Read the model definition and answer for the solid it produces. Units are mm, in the model's axes. A direction names the side the tool comes from. Coordinates: 2 decimals unless noted, no trailing zeros. Order: outer loops, then holes, each group sorted by start corner. A loop starts at its lowest first (then second) coordinate and runs counter-clockwise, first axis right, second up. Notation, with made-up numbers: (49, 27.5) -> (94, 27.5) arc R29 ccw to (94, 53.5) -> close; hole circle Ø10 at (1, 26). An arc over 180 degrees is marked (long way). Use CSV: the item, a comma, the result in double quotes.
```python
from build123d import *

# Parameters (mm, degrees)
SKETCH2_W                   = 38.65
SKETCH2_H                   = 38.65
BOSS_EXTRUDE1_DEPTH         = 1.5875
SKETCH8_W                   = 7.040833333
SKETCH8_H                   = 3.175
BOSS_EXTRUDE3_DEPTH         = 3.175
LPATTERN3_COUNT             = 3
LPATTERN3_PITCH             = 13.941666667
CIRPATTERN1_COUNT           = 4
CIRPATTERN1_COPY_1_SKETCH_W = 7.040833333
CIRPATTERN1_COPY_1_SKETCH_H = 3.175
CIRPATTERN1_COPY_1_DEPTH    = 3.175
CIRPATTERN1_COPY_2_SKETCH_W = 7.040833333
CIRPATTERN1_COPY_2_SKETCH_H = 3.175
CIRPATTERN1_COPY_2_DEPTH    = 3.175
CIRPATTERN1_COPY_3_SKETCH_W = 7.040833333
CIRPATTERN1_COPY_3_SKETCH_H = 3.175
CIRPATTERN1_COPY_3_DEPTH    = 3.175
CIRPATTERN1_COPY_4_SKETCH_W = 7.040833333
CIRPATTERN1_COPY_4_SKETCH_H = 3.175
CIRPATTERN1_COPY_4_DEPTH    = 3.175
CIRPATTERN1_COPY_5_SKETCH_W = 7.040833333
CIRPATTERN1_COPY_5_SKETCH_H = 3.175
CIRPATTERN1_COPY_5_DEPTH    = 3.175
CIRPATTERN1_COPY_6_SKETCH_W = 7.040833333
CIRPATTERN1_COPY_6_SKETCH_H = 3.175
CIRPATTERN1_COPY_6_DEPTH    = 3.175
SKETCH15_R                  = 17.5
CUT_EXTRUDE8_DEPTH          = 32.977814575


with BuildPart() as part:
    # Sketch2 → Boss-Extrude1 (new, symmetric)
    with BuildSketch(Plane(origin=(0, 0, 0), x_dir=(1, 0, 0), z_dir=(0, 1, 0))):
        Rectangle(SKETCH2_W, SKETCH2_H)
    extrude(amount=BOSS_EXTRUDE1_DEPTH, both=True)

    # Sketch8 → Boss-Extrude3 (add)
    with BuildSketch(Plane.ZY.offset(19.325)):
        with Locations((-15.804583334, 0)):
            Rectangle(SKETCH8_W, SKETCH8_H)
    boss_extrude3 = extrude(amount=BOSS_EXTRUDE3_DEPTH)

    # LPattern3: Boss-Extrude3 ×3
    with Locations(*[(0, 0, i * LPATTERN3_PITCH) for i in range(1, LPATTERN3_COUNT)]):
        add(boss_extrude3)

    # CirPattern1: Boss-Extrude3 ×4 about axis
    cirpattern1_axis = Axis((0, 0, 0), (0, 1, 0))
    for i in range(1, CIRPATTERN1_COUNT):
        add(boss_extrude3.rotate(cirpattern1_axis, i * 360 / CIRPATTERN1_COUNT))

    # CirPattern1 copy 1 sketch → CirPattern1 copy 1 (add)
    with BuildSketch(Plane(origin=(13.941666667, 0, 19.325), x_dir=(1, 0, 0), z_dir=(0, 0, 1))):
        with Locations((-15.804583334, 0)):
            Rectangle(CIRPATTERN1_COPY_1_SKETCH_W, CIRPATTERN1_COPY_1_SKETCH_H)
    extrude(amount=CIRPATTERN1_COPY_1_DEPTH)

    # CirPattern1 copy 2 sketch → CirPattern1 copy 2 (add)
    with BuildSketch(Plane(origin=(19.325, 0, -13.941666667), x_dir=(0, 0, -1), z_dir=(1, 0, 0))):
        with Locations((-15.804583334, 0)):
            Rectangle(CIRPATTERN1_COPY_2_SKETCH_W, CIRPATTERN1_COPY_2_SKETCH_H)
    extrude(amount=CIRPATTERN1_COPY_2_DEPTH)

    # CirPattern1 copy 3 sketch → CirPattern1 copy 3 (add)
    with BuildSketch(Plane(origin=(-13.941666667, 0, -19.325), x_dir=(-1, 0, 0), z_dir=(0, 0, -1))):
        with Locations((-15.804583334, 0)):
            Rectangle(CIRPATTERN1_COPY_3_SKETCH_W, CIRPATTERN1_COPY_3_SKETCH_H)
    extrude(amount=CIRPATTERN1_COPY_3_DEPTH)

    # CirPattern1 copy 4 sketch → CirPattern1 copy 4 (add)
    with BuildSketch(Plane(origin=(27.883333333, 0, 19.325), x_dir=(1, 0, 0), z_dir=(0, 0, 1))):
        with Locations((-15.804583334, 0)):
            Rectangle(CIRPATTERN1_COPY_4_SKETCH_W, CIRPATTERN1_COPY_4_SKETCH_H)
    extrude(amount=CIRPATTERN1_COPY_4_DEPTH)

    # CirPattern1 copy 5 sketch → CirPattern1 copy 5 (add)
    with BuildSketch(Plane(origin=(19.325, 0, -27.883333333), x_dir=(0, 0, -1), z_dir=(1, 0, 0))):
        with Locations((-15.804583334, 0)):
            Rectangle(CIRPATTERN1_COPY_5_SKETCH_W, CIRPATTERN1_COPY_5_SKETCH_H)
    extrude(amount=CIRPATTERN1_COPY_5_DEPTH)

    # CirPattern1 copy 6 sketch → CirPattern1 copy 6 (add)
    with BuildSketch(Plane(origin=(-27.883333333, 0, -19.325), x_dir=(-1, 0, 0), z_dir=(0, 0, -1))):
        with Locations((-15.804583334, 0)):
            Rectangle(CIRPATTERN1_COPY_6_SKETCH_W, CIRPATTERN1_COPY_6_SKETCH_H)
    extrude(amount=CIRPATTERN1_COPY_6_DEPTH)

    # Sketch15 → Cut-Extrude8 (cut, through all)
    with BuildSketch(Plane(origin=(0, 1.5875, 0), x_dir=(1, 0, 0), z_dir=(0, 1, 0))):
        with Locations(Location((0, 0, 0), (0, 0, 270))):
            Circle(SKETCH15_R)
    extrude(amount=-CUT_EXTRUDE8_DEPTH, mode=Mode.SUBTRACT)


solid = part.part
```
Item 1: Find section B-B, the plane z = 0. Give the vertices of the cut face in (x, y).
Return value:
outline,"(-22.5, -1.59) -> (-17.5, -1.59) -> (-17.5, 1.59) -> (-22.5, 1.59) -> close; (17.5, -1.59) -> (22.5, -1.59) -> (22.5, 1.59) -> (17.5, 1.59) -> close"
Item 2: Straight lines are drawn through the part: line 1 along X through (y, z) = (0.7, -20) (1 decimal); line 2 along X through (y, z) = (0.7, 0); line 3 along Z through (x, y) = (-3, -0.85) (3 decimals). For each, find the intervals that lie inside material, in ascending order.
Return value:
line 1,"x = -15.6 to -8.6, -1.7 to 5.4, 12.3 to 19.3"
line 2,"x = -22.5 to -17.5, 17.5 to 22.5"
line 3,"z = -19.325 to -17.241, 17.241 to 22.5"
Item 3: The mould has two halves that part along X. Classify faces 6 (the flat face through (21, 0, 5.383)), 7 (the flat face through (-22.5, 0, 12)), 8 (the flat face through (-12.284, 0, 21)), 9 (the flat face through (19.325, 0, 9)): +X half, -X half, draft (parallel to the pull), parting line (faces both ways), or undercut.
Return value:
face 6,"draft"
face 7,"-X half"
face 8,"undercut"
face 9,"+X half"
Item 4: Find section A-A, the plane x = 0. Give the vertices of the cut face in (y, z), then the cut area to 4 significant figures.
Return value:
outline,"(-1.59, -22.5) -> (1.59, -22.5) -> (1.59, -17.5) -> (-1.59, -17.5) -> close; (-1.59, 17.5) -> (1.59, 17.5) -> (1.59, 22.5) -> (-1.59, 22.5) -> close"
area,"31.75 mm^2"
Item 5: A tool of negligible diameter and unlimited length cuts with its end or side. For faces 1 (the flat face through (21, 0, -1.657)), 2 (the flat face through (-21, 0, 1.657)), 3 (the flat face through (8.558, 0, 21)), 4 (the flat face through (5.383, 0, -21)), 5 (the flat face through (19.325, 0, -19)), from which of +Z, -Z, +X, -X, +Y, -Y can it reach the whole face along a straight path? Write none if from no direction.
Return value:
face 1,"+X, +Y, -Y"
face 2,"-X, +Y, -Y"
face 3,"+Z, +Y, -Y"
face 4,"-Z, +Y, -Y"
face 5,"-Z, +X, +Y, -Y"
Item 6: Each of these flat-tipped pins is pushed along its axis until it touches: P1, Ø1, axis at y = 0, z = 20, coming from the +X side; P2, Ø1.6, axis at y = 0, z = -21.5, coming from the +X side (3 decimals); P3, Ø1, axis at x = -20.5, y = 0, coming from the -Z side (3 decimals). Where does it stop, or does it pass through?
Return value:
P1,"stops at x = 15.6"
P2,"stops at x = 19.325"
P3,"stops at z = -19.325"
